CAD build for the part. Positions are in the model's coordinates, mm. Face numbers are marked on the shaded views. A direction names the side the tool comes from. Round coordinates to 2 decimals unless told otherwise and drop trailing zeros. Write each loop counter-clockwise with the first axis right and the second up, starting at its lowest first coordinate (ties: lowest second). Pieces come first, ordered by that corner, then holes. Notation, with made-up numbers: (-31.75, 51.25) -> (2.25, 51.25) arc R28 cw to (2.25, 86.25) -> close; hole circle Ø2 at (-15, 33). An arc over 180 degrees is marked (long way). Put each result on its own line as item: value. Start each with the question number.
1. 3-axis set-ups, long thin cutter, end or side, ignore diameter. For the marked faces 1, 2 and 3: which of +Z, -Z, +X, -X, +Y, -Y reach the whole face in a straight line?
2. Saw through at A-A on z = -3.25. List the corners of the cut face in (x, y).
3. Flat gauge pins, fed straight in: P1, Ø1.5, axis at x = -13.5, z = 3, coming from the -Y side; P2, Ø2.5, axis at y = 52.5, z = -1, coming from the -X side; P3, Ø4, axis at y = 3.2, z = 0, coming from the -X side; P4, Ø0.8, axis at x = -37.5, z = 0.5, coming from the +Y side. Where does each tip first touch, or does it go through?
4. Saw through at B-B on y = 3.2. List the corners of the cut face in (x, z) (3 decimals).
5. Drill centre lines: line 1 (Z direction, x = -15.35, y = 3.2) (3 decimals); line 2 (Y direction, x = -19.2, z = 0); line 3 (Z direction, x = -18.6, y = 3.2). Where is each one in solid material? Low to high. Write a range as from..to.
6. Saw through at C-C on x = -29. List the corners of the cut face in (y, z), and give its area (3 significant figures).
7. Saw through at D-D on y = 42. List the corners of the cut face in (x, z).
8. Pull direction Y, two halves, no side cores. Call the marked faces 4, 5, 6 and 7: pulls with the +Y half, pulls with the -Y half, needs draft (parallel to the pull), parting line crosses it, or undercut.
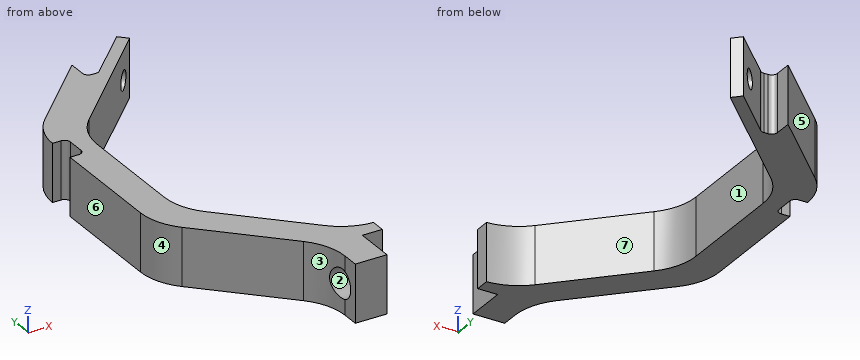
from build123d import *

# Parameters (mm, degrees)
ESTRUSIONE_ESTRUSIONE1_DEPTH = 5
SCHIZZO2_R                   = 2.5
TAGLIO_ESTRUSIONE2_DEPTH     = 3.5
SCHIZZO3_R                   = 1.625
TAGLIO_ESTRUSIONE3_DEPTH     = 10
RACCORDO1_R                  = 10
SCHIZZO4_W                   = 2.5
SCHIZZO4_H                   = 5
TAGLIO_ESTRUSIONE4_DEPTH     = 10
RACCORDO2_R                  = 1
SCHIZZO5_R                   = 1.625
TAGLIO_ESTRUSIONE5_DEPTH     = 10


with BuildPart() as part:
    # Schizzo1 → Estrusione-Estrusione1 (new, symmetric)
    with BuildSketch(Plane.XY):
        Polygon((-13.891157033, -0.6), (-19.391157033, -0.6), (-19.391157033, 6.4), (-38.302699765, 25.311542732), (-38.302699765, 58.4), (-23.302699765, 73.4), (-23.302699765, 69.4), (-21.131126889, 69.4), (-13.131126889, 77.4), (-11.716913327, 75.985786438), (-32.802699765, 54.9), (-32.802699765, 27.589717325), (-14.11298244, 8.9), (-10.427699765, 8.9), (-10.427699765, 6.4), (-13.891157033, 6.4), align=None)
    extrude(amount=ESTRUSIONE_ESTRUSIONE1_DEPTH, both=True)

    # Schizzo2 → Taglio-Estrusione2 (cut)
    with BuildSketch(Plane.ZY.offset(19.391157033)):
        with Locations(Location((0, 3.2, 0), (0, 0, 270))):
            Circle(SCHIZZO2_R)
    extrude(amount=-TAGLIO_ESTRUSIONE2_DEPTH, mode=Mode.SUBTRACT)

    # Schizzo3 → Taglio-Estrusione3 (cut)
    with BuildSketch(Plane.ZY.offset(19.391157033)):
        with Locations(Location((0, 3.2, 0), (0, 0, 270))):
            Circle(SCHIZZO3_R)
    extrude(amount=-TAGLIO_ESTRUSIONE3_DEPTH, mode=Mode.SUBTRACT)

    # Raccordo1
    # the kernel refuses this fillet: 10 mm, written as the material it adds along each edge
    with BuildSketch(Plane(origin=(-19.391157033, 6.4, 5), x_dir=(0, -1, 0), z_dir=(0, 0, -1))) as raccordo1_piece_1_section:
        with BuildLine():
            CenterArc((RACCORDO1_R * 0.414213562373, RACCORDO1_R), RACCORDO1_R, 225, 45)
            Line((-RACCORDO1_R * 0.292893218813, RACCORDO1_R * 0.292893218813), (0, 0))
            Line((0, 0), (RACCORDO1_R * 0.414213562373, 0))
        make_face()
    raccordo1_piece_1 = extrude(amount=10, mode=Mode.PRIVATE)
    raccordo1_piece_1 = raccordo1_piece_1 - Plane(origin=(-19.391157033, 3.2, 0), x_dir=(0, -1, 0), z_dir=(-1, 0, 0)) * Cylinder(2.5, 37, mode=Mode.PRIVATE)
    add(raccordo1_piece_1)
    with BuildSketch(Plane(origin=(-14.11298244, 8.9, 5), x_dir=(-0.7071067811865495, 0.7071067811865456, 0), z_dir=(0, 0, -1))) as raccordo1_piece_2:
        with BuildLine():
            CenterArc((4.126652993, 10), RACCORDO1_R, 227.681279823, 42.318720177)
            Line((-2.60588837, 2.60588837), (0, 0))
            Line((0, 0), (4.126652993, 0))
        make_face()
    extrude(amount=10)
    with BuildSketch(Plane(origin=(-32.802699765, 27.589717325, 5), x_dir=(0, 1, 0), z_dir=(0, 0, -1)), Plane(origin=(-32.802699765, 54.9, 5), x_dir=(0.7071067811865458, 0.7071067811865492, 0), z_dir=(0, 0, -1))) as raccordo1_piece_3:
        with BuildLine():
            CenterArc((RACCORDO1_R * 0.414213562373, RACCORDO1_R), RACCORDO1_R, 225, 45)
            Line((-RACCORDO1_R * 0.292893218813, RACCORDO1_R * 0.292893218813), (0, 0))
            Line((0, 0), (RACCORDO1_R * 0.414213562373, 0))
        make_face()
    extrude(amount=10)
    # the kernel refuses this fillet: 10 mm, written as the material it takes off along each edge
    with BuildSketch(Plane(origin=(-38.302699765, 25.311542732, 15.355339059), x_dir=(0.7071067811865497, -0.7071067811865454, 0), z_dir=(0, 0, -1)), Plane(origin=(-38.302699765, 58.4, 15.355339059), x_dir=(0, -1, 0), z_dir=(0, 0, -1))) as raccordo1_2_piece_1:
        with BuildLine():
            CenterArc((RACCORDO1_R * 0.414213562373, -RACCORDO1_R), RACCORDO1_R, 90, 45)
            Line((-RACCORDO1_R * 0.292893218813, -RACCORDO1_R * 0.292893218813), (0, 0))
            Line((0, 0), (RACCORDO1_R * 0.414213562373, 0))
        make_face()
    extrude(amount=30.710678119, mode=Mode.SUBTRACT)

    # Schizzo4 → Taglio-Estrusione4 (cut)
    with BuildSketch(Plane(origin=(0, 0, -5), x_dir=(-1, 0, 0), z_dir=(0, 0, -1))):
        with Locations((37.052699765, 51.9)):
            Rectangle(SCHIZZO4_W, SCHIZZO4_H)
    extrude(amount=-TAGLIO_ESTRUSIONE4_DEPTH, mode=Mode.SUBTRACT)

    # Raccordo2
    raccordo2_edges = [part.edges().sort_by_distance(p)[0] for p in [
        (-35.802699765, 49.4, 0),
        (-35.802699765, 54.4, 0),
        (-23.302699765, 69.4, 0),
        (-21.131126889, 69.4, 0),
    ]]
    fillet(raccordo2_edges, radius=RACCORDO2_R)

    # Schizzo5 → Taglio-Estrusione5 (cut)
    with BuildSketch(Plane(origin=(-43.851349882, 43.851349882, 0), x_dir=(0, 0, -1), z_dir=(0.707106781186549, -0.707106781186546, 0))):
        with Locations(Location((0, 41.444955996, 0), (0, 0, 90))):
            Circle(SCHIZZO5_R)
    extrude(amount=-TAGLIO_ESTRUSIONE5_DEPTH, mode=Mode.SUBTRACT)


solid = part.part
Return value:
1. face 1: +Z, -Z, +X
1. face 2: -X
1. face 3: +Z, -Z, -X, -Y
2. outline: (-38.3, 29.45) arc R10 ccw to (-35.37, 22.38) -> (-22.32, 9.33) arc R10 cw to (-19.39, 2.26) -> (-19.39, -0.6) -> (-13.89, -0.6) -> (-13.89, 6.4) -> (-10.43, 6.4) -> (-10.43, 8.9) arc R10 cw to (-17.03, 11.82) -> (-29.87, 24.66) arc R10 cw to (-32.8, 31.73) -> (-32.8, 50.76) arc R10 cw to (-29.87, 57.83) -> (-11.72, 75.99) -> (-13.13, 77.4) -> (-20.84, 69.69) arc R1 cw to (-21.55, 69.4) -> (-22.3, 69.4) arc R1 cw to (-23.3, 70.4) -> (-23.3, 73.4) -> (-35.37, 61.33) arc R10 ccw to (-38.3, 54.4) -> (-36.8, 54.4) arc R1 cw to (-35.8, 53.4) -> (-35.8, 50.4) arc R1 cw to (-36.8, 49.4) -> (-38.3, 49.4) -> close
3. P1: stops at y = -0.6
3. P2: stops at x = -35.87
3. P3: stops at x = -15.89
3. P4: stops at y = 59.01
4. outline: (-19.436, -5) -> (-13.891, -5) -> (-13.891, -1.625) -> (-15.891, -1.625) -> (-15.891, -2.5) -> (-19.436, -2.5) -> close; (-19.436, 2.5) -> (-15.891, 2.5) -> (-15.891, 1.625) -> (-13.891, 1.625) -> (-13.891, 5) -> (-19.436, 5) -> close
5. line 1: z = -5..-1.625, 1.625..5
5. line 2: y = -0.6..0.7, 5.7..13.99, 68.5..71.33
5. line 3: z = -5..-2.5, 2.5..5
6. outline: (16.01, -5) -> (23.79, -5) -> (23.79, 5) -> (16.01, 5) -> close; (58.7, -5) -> (67.7, -5) -> (67.7, 5) -> (58.7, 5) -> close
6. area: 168 mm^2
7. outline: (-38.3, -5) -> (-32.8, -5) -> (-32.8, 5) -> (-38.3, 5) -> close
8. face 4: pulls with the -Y half
8. face 5: pulls with the +Y half
8. face 6: needs draft
8. face 7: undercut
